Can you work these out from the model? Positions are in its coordinate system, mm. Coordinates: 2 decimals unless noted, no trailing zeros. Order: outer loops, then holes, each group sorted by start corner. A loop starts at its lowest first (then second) coordinate and runs counter-clockwise, first axis right, second up. Notation, with made-up numbers: M 71,1.25 L 103,1.25 A35 cw 103,34.25 Z; hole C 27.25,7.25 d10. An arc over 180 degrees is marked long. Answer as CSV lines item,"result". Start each with the question number.
1. If we section it at D-D (z = 19.5): List the corners of the cut face in (x, y) for me.
2. I need wall thicknesses on line 1 along Y through (x, z) = (-0.5, 0); line 2 along Z through (x, y) = (7.75, 0); line 3 along Z through (x, y) = (-6, 0). Which ranges of each line are inside material? Lowest first, please. Write a range as from..to.
3. Will these pins go through, and if not, where does the flat tip stop? pin 1 (6 mm diameter, centred on y = -10, z = -3.5, fed in from +X); pin 2 (1.5 mm diameter, centred on y = -3, z = 32, fed in from -X); pin 3 (6 mm diameter, centred on x = 5.5, z = 50, fed in from +Y).
4. If we section it at A-A (z = 0): List the corners of the cut face in (x, y) for me.
5. If we mould it in two halves opening along Y, with no side actions, what happens to faces 1 (the face through (3, 4, 37)), 2 (the face through (0, 0, 60)), 3 (the face through (0.16, -1.08, -4.88))? For each: released by +Y, released by -Y, zero draft, split by the parting line, or undercut.
6. If we section it at B-B (x = -8.75): List the corners of the cut face in (y, z) for me.
7. If we section it at C-C (y = 8.25): List the corners of the cut face in (x, z) for me.
```python
from build123d import *

# Parameters (mm, degrees)
F3_R     = 5
F4_DEPTH = 60
F2_R     = 5
F5_DEPTH = 15000
F6_R     = 5


with BuildPart() as f1:
    # F0 (on Right) → F1 (revolve)
    with BuildSketch(Plane.YZ):
        with BuildLine():
            Line((0, 12.5), (0, -12.5))
            ThreePointArc((0, -12.5), (12.5, 0), (0, 12.5))
        make_face()
    revolve(axis=Axis((0, 0, -1.2070862576), (0, 0, -1)))

    # F3 (on Top) → F4 (join)
    with BuildSketch(Plane.XY):
        Circle(F3_R)
    extrude(amount=F4_DEPTH)

    # F2 (on Right) → F5 (cut, symmetric)
    with BuildSketch(Plane.YZ):
        Circle(F2_R)
    extrude(amount=F5_DEPTH, both=True, mode=Mode.SUBTRACT)

    # F6
    f6_edges = [f1.edges().sort_by_distance(p)[0] for p in [
        (3.535534, 3.535534, 11.456439),
        (-3.535534, -3.535534, 11.456439),
    ]]
    fillet(f6_edges, radius=F6_R)


solid = f1.part
```
Solved:
1,outline,"C 0,0 d10"
2,line 1,"-12.49..-5, 5..12.49"
2,line 2,"-9.81..-5, 5..9.81"
2,line 3,"-10.97..-5, 5..11.36"
3,pin 1,"x = 9.93"
3,pin 2,"x = -4.47"
3,pin 3,"y = 4.33"
4,outline,"M -11.46,-5 A12.5 ccw 11.46,-5 Z; M -11.46,5 L 11.46,5 A12.5 ccw Z"
5,face 1,"split by the parting line"
5,face 2,"zero draft"
5,face 3,"undercut"
6,outline,"C 0,0 d17.85; hole C 0,0 d10"
7,outline,"C 0,0 d18.78"
